from build123d import *

# Parameters (mm, degrees)
SKETCH1_R           = 2
BOSS_EXTRUDE1_DEPTH = 14.5
CUT_EXTRUDE1_START  = -8
CUT_EXTRUDE1_DEPTH  = 8
CHAMFER1_SIZE       = 0.1


with BuildPart() as part:
    # Sketch1 → Boss-Extrude1 (new body)
    with BuildSketch(Plane.XY):
        with Locations(Location((0, 0, 0), (0, 0, 180))):
            Circle(SKETCH1_R)
    extrude(amount=BOSS_EXTRUDE1_DEPTH)

    # Sketch2 → Cut-Extrude1 (cut)
    with BuildSketch(Plane.XY.offset(14.5).offset(CUT_EXTRUDE1_START)):
        with BuildLine():
            Line((-1.322875656, 1.5), (1.322875656, 1.5))
            ThreePointArc((1.322875656, 1.5), (0, 2), (-1.322875656, 1.5))
        make_face()
    extrude(amount=CUT_EXTRUDE1_DEPTH, mode=Mode.SUBTRACT)

    # Chamfer1
    chamfer1_edges = [part.edges().sort_by_distance(p)[0] for p in [
        (0.822875656, -1.822875656, 14.5),
    ]]
    chamfer(chamfer1_edges, length=CHAMFER1_SIZE)


solid = part.part
Part model, mm, in its own coordinate system. A direction names the side the tool comes from. Give positions to 0.01 mm unless a question says otherwise; leave off trailing zeros. Loops run counter-clockwise (first coordinate to the right, second up) from the corner with the lowest first, then second, coordinate; pieces in that order, holes last. Notation, with made-up numbers: M 80.25,89 L 104.25,89 A13 cw 104.25,114 Z; hole C -1.75,81 d2. An arc over 180 degrees is marked long. Put each result on its own line as item: value. Start each with the question number.
1) Flat gauge pin, fed straight in: pin 1 (1.3 mm diameter, centred on x = 0, z = 10.5, fed in from +Y). Where does the tip first touch, or does it go through?
2) 3-axis set-ups, long thin cutter, end or side, ignore diameter. For faces 1 (the flat face through (0, 1.5, 10)), 2 (the flat face through (0, 0, 14.5)): which of +Z, -Z, +X, -X, +Y, -Y reach the whole face in a straight line?
3) Saw through at B-B (z = 3.5). List the corners of the cut face in (x, y).
4) Probe probe 1 along X at (y, z) = (-1.5, 3.25); probe 2 along X at (y, z) = (0.1, 13.25); probe 3 along Y at (x, z) = (-0.05, 7.25). List the from-to ranges inside material, lowest first.
5) Saw through at C-C (z = 13). List the corners of the cut face in (x, y), then the cut area to 3 significant figures.
6) Saw through at A-A (x = 0). List the corners of the cut face in (y, z), then the cut area to 3 significant figures.
Numbers:
1. pin 1: y = 1.5
2. face 1: +Z, +X, -X, +Y
2. face 2: +Z, +X, -X, +Y, -Y
3. outline: C 0,0 d4
4. probe 1: -1.32 to 1.32
4. probe 2: -2 to 2
4. probe 3: -2 to 1.5
5. outline: M -1.32,1.5 A2 ccw long 1.32,1.5 Z
5. area: 11.7 mm^2
6. outline: M -2,0 L 2,0 L 2,6.5 L 1.5,6.5 L 1.5,14.5 L -1.9,14.5 L -2,14.4 Z
6. area: 54.0 mm^2
